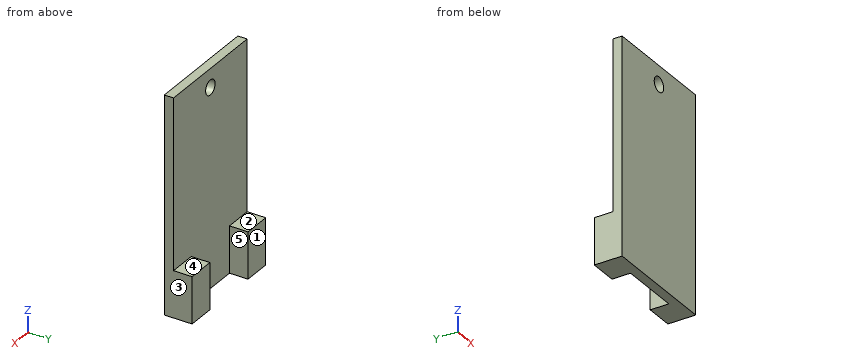
Autodesk Inventor part; units mm, degrees
ref_plane "YZ Plane" through (0, 0, 0) normal (1, 0, 0) x (0, 1, 0)
ref_plane "XZ Plane" through (0, 0, 0) normal (0, 1, 0) x (-1, 0, 0)
ref_plane "XY Plane" through (0, 0, 0) normal (0, 0, 1) x (1, 0, 0)
sketch "Sketch1" plane through (0, 0, 0) normal (0, 1, 0) x (-1, 0, 0)
  line L0 (0, 0) -> (-25, 0)
  line L1 (-25, 0) -> (-25, -46.5)
  line L2 (-25, -46.5) -> (0, -46.5)
  line L3 (0, -46.5) -> (0, 0)
  dimension "d0" = 25
  dimension "d1" = 46.5
extrude "Extrusion1" add sketch "Sketch1" along normal blind 2
sketch "Sketch2" plane through (0, 2, 0) normal (0, 1, 0) x (1, 0, 0)
  line L0 (25, 46.5) -> (0, 46.5)
  line L1 (0, 46.5) -> (6, 46.5)
  line L2 (6, 46.5) -> (6, 36.5)
  line L3 (6, 36.5) -> (0, 36.5)
  line L4 (0, 36.5) -> (0, 46.5)
  line L5 (25, 46.5) -> (19, 46.5)
  line L6 (19, 46.5) -> (19, 36.5)
  line L7 (19, 36.5) -> (25, 36.5)
  line L8 (25, 36.5) -> (25, 46.5)
  point P0 (0, 0)
  dimension "d4" = 6
  dimension "d5" = 10
  dimension "d6" = 6
extrude "Extrusion2" add sketch "Sketch2" along normal blind 4
sketch "Sketch4" plane through (0, 2, 0) normal (0, 1, 0) x (1, 0, 0)
  line L0 (0, 0) -> (25, 0)
  line L1 (25, 0) -> (25, 36.5)
  point P0 (12.5, 4)
  dimension "d18" = 4
  dimension "d19" = 12.5
hole "Hole2" at (12.5, 2, -4) direction (0, -1, 0) diameter 3.2 end through all
properties part number "mlx_mount_4mm"
Part model, mm, in its own coordinate system. Face numbers are marked on the shaded views. A direction names the side the tool comes from. Give positions to 0.01 mm unless a question says otherwise; leave off trailing zeros. Order: outer loops, then holes, each group sorted by start corner. A loop starts at its lowest first (then second) coordinate and runs counter-clockwise, first axis right, second up. Notation, with made-up numbers: (67, 39.25) - (115, 39.25) arc R35 cw to (115, 71.25) - close; hole circle Ø2 at (-12.5, 53). An arc over 180 degrees is marked (long way). Use one line per item in the form item = value.
Item 1: Slice it at B-B on z = -4. Give the cut face in (x, y).
Solution:
outline = (0, 0) - (10.9, 0) - (10.9, 2) - (0, 2) - close; (14.1, 0) - (25, 0) - (25, 2) - (14.1, 2) - close
Item 2: Two-plate mould, pull along X, no slides. Class the marked faces 3, 4 and 5: released by +X, released by -X, zero draft, split by the parting line, or undercut.
Solution:
face_3 = released by +X
face_4 = zero draft
face_5 = undercut
Item 3: Probe probe 1 along X at (y, z) = (1.45, -4); probe 2 along Z at (x, y) = (12.5, 0.8); probe 3 along Y at (x, z) = (9.5, -13.5). List the from-to ranges inside material, lowest first. Write a range as from..to.
Solution:
probe_1 = 0..10.9, 14.1..25
probe_2 = -46.5..-5.6, -2.4..0
probe_3 = 0..2
Item 4: Which spindle directions (+Z, -Z, +X, -X, +Y, -Y) get a long thin tool onto all of the face, cutting with end or side? Do the marked faces 1 and 2. Say none if no direction does.
Solution:
face_1 = +Z, -Z, +X, -X, +Y
face_2 = +Z, +X, -X, +Y
Item 5: Slice it at A-A on y = 4.85. Give the cut face in (x, z), and give its area (3 significant figures).
Solution:
outline = (0, -46.5) - (6, -46.5) - (6, -36.5) - (0, -36.5) - close; (19, -46.5) - (25, -46.5) - (25, -36.5) - (19, -36.5) - close
area = 120 mm2
Item 6: Slice it at C-C on x = 4.25. Give the cut face in (y, z), and give its area (3 significant figures).
Solution:
outline = (0, -46.5) - (6, -46.5) - (6, -36.5) - (2, -36.5) - (2, 0) - (0, 0) - close
area = 133 mm2
Item 7: Slice it at D-D on z = -42.5. Give the cut face in (x, y).
Solution:
outline = (0, 0) - (25, 0) - (25, 6) - (19, 6) - (19, 2) - (6, 2) - (6, 6) - (0, 6) - close
Item 8: Pin check, flat tip, straight feed: pin 1 Ø3 at (x, z) = (10.5, -10.5) entering from +Y. Stop position of the tip, or through.
Solution:
pin_1 = 2
